Verification items for the finished model (mm, model axes). Face numbers are marked on the shaded views. A direction names the side the tool comes from. Round coordinates to 2 decimals unless told otherwise and drop trailing zeros. Loops run counter-clockwise (first coordinate to the right, second up) from the corner with the lowest first, then second, coordinate; pieces in that order, holes last. Notation, with made-up numbers: (57, 34) -> (111, 34) arc R21 cw to (111, 45) -> close; hole circle Ø5 at (9.25, 7). An arc over 180 degrees is marked (long way). Use CSV: the item, a comma, the result in double quotes. Start each with the question number.
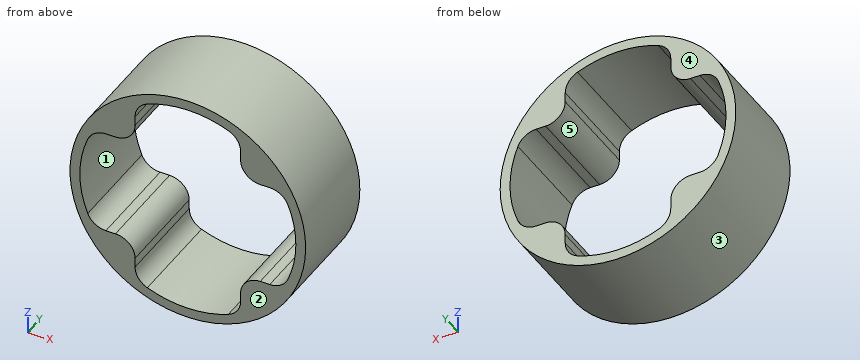
```python
from build123d import *

# Parameters (mm, degrees)
F0_R     = 30
F0_R_2   = 27.5
F1_DEPTH = 25
F3_DEPTH = 25
F4_R     = 5


with BuildPart() as f1:
    # F0 (on Front) → F1 (new body)
    with BuildSketch(Plane.XZ):
        Circle(F0_R)
        Circle(F0_R_2, mode=Mode.SUBTRACT)
    extrude(amount=F1_DEPTH)

    # F2 (on Front) → F3 (join)
    with BuildSketch(Plane.XZ):
        with BuildLine():
            Line((-24.4350288425, 13.4350288425), (-18.4350288425, 13.4350288425))
            ThreePointArc((-18.4350288425, 13.4350288425), (-14.8994949366, 14.8994949366), (-13.4350288425, 18.4350288425))
            Line((-13.4350288425, 18.4350288425), (-13.4350288425, 24.4350288425))
            ThreePointArc((-13.4350288425, 24.4350288425), (-19.7176397489, 19.7176397489), (-24.4350288425, 13.4350288425))
        make_face()
        with BuildLine():
            ThreePointArc((18.4350288425, -13.4350288425), (14.8994949366, -14.8994949366), (13.4350288425, -18.4350288425))
            Line((13.4350288425, -18.4350288425), (13.4350288425, -24.4350288425))
            ThreePointArc((13.4350288425, -24.4350288425), (19.7176397489, -19.7176397489), (24.4350288425, -13.4350288425))
            Line((24.4350288425, -13.4350288425), (18.4350288425, -13.4350288425))
        make_face()
        with BuildLine():
            ThreePointArc((13.4350288425, 18.4350288425), (14.8994949366, 14.8994949366), (18.4350288425, 13.4350288425))
            Line((18.4350288425, 13.4350288425), (24.4350288425, 13.4350288425))
            ThreePointArc((24.4350288425, 13.4350288425), (19.7176397489, 19.7176397489), (13.4350288425, 24.4350288425))
            Line((13.4350288425, 24.4350288425), (13.4350288425, 18.4350288425))
        make_face()
        with BuildLine():
            Line((-13.4350288425, -24.4350288425), (-13.4350288425, -18.4350288425))
            ThreePointArc((-13.4350288425, -18.4350288425), (-14.8994949366, -14.8994949366), (-18.4350288425, -13.4350288425))
            Line((-18.4350288425, -13.4350288425), (-24.4350288425, -13.4350288425))
            ThreePointArc((-24.4350288425, -13.4350288425), (-19.7176397489, -19.7176397489), (-13.4350288425, -24.4350288425))
        make_face()
    extrude(amount=F3_DEPTH)

    # F4
    f4_edges = [f1.edges().sort_by_distance(p)[0] for p in [
        (-13.435029, -12.5, 23.994791),
        (-23.994791, -12.5, 13.435029),
        (-23.994791, -12.5, -13.435029),
        (-13.435029, -12.5, -23.994791),
        (13.435029, -12.5, 23.994791),
        (23.994791, -12.5, 13.435029),
        (13.435029, -12.5, -23.994791),
        (23.994791, -12.5, -13.435029),
    ]]
    fillet(f4_edges, radius=F4_R)


solid = f1.part
```
Q1. Release check for a two-part mould opening along X. For the marked faces 1, 2 and 3 record: +X half, -X half, draft (parallel to the pull), parting line (faces both ways), or undercut.
Q2. Cross-section at C-C (x = -24). Record the boundary of the cut face in (y, z).
Q3. Cross-section at A-A (y = -12.5). Record the boundary of the cut face in (x, z), and give its area (3 significant figures).
Q4. Depth check by flat-ended pin: pin 1 Ø1.2 at (x, y) = (-19.5, -18.5) entering from -Z; pin 2 Ø10 at (y, z) = (-13, 6) entering from +X; pin 3 Ø1.2 at (x, y) = (19, -16.5) entering from +Z. Enter the tip coordinate at first touch or a pass-through.
Q5. Tool access check on the marked faces 4 and 5. Record the directions out of +Z, -Z, +X, -X, +Y, -Y that give a thin tool (end or side, any length) a straight path to the whole face; none if there is none.
Q6. Thickness scan on L1, parallel to X at y = -4.25, z = -0.5; L2, parallel to X at y = -23, z = 12; L3, parallel to Z at x = -3.5, y = -5. Record the ranges inside material, lowest first. Write a range as from..to.
Q7. Cross-section at B-B (z = 0). Record the boundary of the cut face in (x, y).
Answer list:
1,face 1,"undercut"
1,face 2,"draft"
1,face 3,"parting line"
2,outline,"(-25, -18) -> (0, -18) -> (0, -12.33) -> (-25, -12.33) -> close; (-25, 12.33) -> (0, 12.33) -> (0, 18) -> (-25, 18) -> close"
3,outline,"circle Ø60 at (0, 0); hole (-25.49, -10.31) arc R5 ccw to (-20.86, -13.44) -> (-18.44, -13.44) arc R5 cw to (-13.44, -18.44) -> (-13.44, -20.86) arc R5 ccw to (-10.31, -25.49) arc R27.5 ccw to (10.31, -25.49) arc R5 ccw to (13.44, -20.86) -> (13.44, -18.44) arc R5 cw to (18.44, -13.44) -> (20.86, -13.44) arc R5 ccw to (25.49, -10.31) arc R27.5 ccw to (25.49, 10.31) arc R5 ccw to (20.86, 13.44) -> (18.44, 13.44) arc R5 cw to (13.44, 18.44) -> (13.44, 20.86) arc R5 ccw to (10.31, 25.49) arc R27.5 ccw to (-10.31, 25.49) arc R5 ccw to (-13.44, 20.86) -> (-13.44, 18.44) arc R5 cw to (-18.44, 13.44) -> (-20.86, 13.44) arc R5 ccw to (-25.49, 10.31) arc R27.5 ccw to start"
3,area,"709 mm2"
4,pin 1,"stops at z = -23.3"
4,pin 2,"stops at x = 29.98"
4,pin 3,"stops at z = 23.69"
5,face 4,"+Z, -Z, +X, -X, +Y"
5,face 5,"+Y, -Y"
6,L1,"x = -30..-27.5, 27.5..30"
6,L2,"x = -27.5..-24.36, 24.36..27.5"
6,L3,"z = -29.8..-27.28, 27.28..29.8"
7,outline,"(-30, -25) -> (-27.5, -25) -> (-27.5, 0) -> (-30, 0) -> close; (27.5, -25) -> (30, -25) -> (30, 0) -> (27.5, 0) -> close"
